Input: part model. Units: mm. Frame: model coordinates. A direction names the side the tool comes from. Coordinates: 2 decimals unless noted, no trailing zeros. Order: outer loops, then holes, each group sorted by start corner. A loop starts at its lowest first (then second) coordinate and runs counter-clockwise, first axis right, second up.
from build123d import *

# Parameters (mm, degrees)
BOSS_EXTRUDE1_DEPTH = 48.12
SKETCH3_W           = 16
SKETCH3_H           = 28.73
CUT_EXTRUDE1_DEPTH  = 47.12
SKETCH4_W           = 0.5
SKETCH4_H           = 10
BOSS_EXTRUDE2_DEPTH = 3
SKETCH5_W           = 2
SKETCH5_H           = 22.73
BOSS_EXTRUDE3_DEPTH = 4
SKETCH6_W           = 1
SKETCH6_H           = 19.230578804
CUT_EXTRUDE2_DEPTH  = 1
FILLET1_R           = 1
FILLET2_R           = 1
FILLET3_R           = 1
FILLET4_R           = 1


with BuildPart() as part:
    # Sketch2 → Boss-Extrude1 (new body)
    with BuildSketch(Plane(origin=(0, 0, 0), x_dir=(0, 0, -1), z_dir=(1, 0, 0))):
        Polygon((-1238.520696333, 790.685360665), (-1238.520696333, 788.685360665), (-1221.520696333, 788.685360665), (-1221.520696333, 759.955360665), (-1238.520696333, 759.955360665), (-1238.520696333, 757.955360665), (-1240.520696333, 757.955360665), (-1240.520696333, 790.685360665), align=None)
    extrude(amount=-BOSS_EXTRUDE1_DEPTH)

    # Sketch3 → Cut-Extrude1 (cut)
    with BuildSketch(Plane.ZY.offset(48.12)):
        with Locations((1230.520696333, 774.320360665)):
            Rectangle(SKETCH3_W, SKETCH3_H)
    extrude(amount=-CUT_EXTRUDE1_DEPTH, mode=Mode.SUBTRACT)

    # Sketch4 → Boss-Extrude2 (add)
    with BuildSketch(Plane.ZY.offset(48.12)):
        with Locations((1222.270696333, 774.320360665)):
            Rectangle(SKETCH4_W, SKETCH4_H)
    extrude(amount=BOSS_EXTRUDE2_DEPTH)

    # Sketch5 → Boss-Extrude3 (add)
    with BuildSketch(Plane(origin=(0, 0, 0), x_dir=(0, 0, -1), z_dir=(1, 0, 0))):
        with Locations((-1238.520696333, 774.320360665)):
            Rectangle(SKETCH5_W, SKETCH5_H)
    extrude(amount=BOSS_EXTRUDE3_DEPTH)

    # Sketch6 → Cut-Extrude2 (cut)
    with BuildSketch(Plane.XY.offset(1239.520696333)):
        with Locations((2, 773.582614675)):
            Rectangle(SKETCH6_W, SKETCH6_H)
    extrude(amount=-CUT_EXTRUDE2_DEPTH, mode=Mode.SUBTRACT)

    # Fillet1
    fillet1_edges = [part.edges().sort_by_distance(p)[0] for p in [
        (0, 774.320360665, 1239.520696333),
    ]]
    fillet(fillet1_edges, radius=FILLET1_R - 0.0001)  # a hair under: the kernel refuses the full size

    # Fillet2
    fillet2_edges = [part.edges().sort_by_distance(p)[0] for p in [
        (0, 774.320360665, 1237.520696333),
    ]]
    fillet(fillet2_edges, radius=FILLET2_R)

    # Fillet3
    fillet3_edges = [part.edges().sort_by_distance(p)[0] for p in [
        (0, 785.685360665, 1238.520646333),
    ]]
    fillet(fillet3_edges, radius=FILLET3_R)

    # Fillet4
    fillet4_edges = [part.edges().sort_by_distance(p)[0] for p in [
        (0, 762.955360665, 1238.520646333),
    ]]
    fillet(fillet4_edges, radius=FILLET4_R)


solid = part.part
Item 1: Ray query, probe 1 along Z at (x, y) = (-27, 769.5); probe 2 along Z at (x, y) = (-3, 759); probe 3 along X at (y, z) = (777, 1227.25). Return the intervals inside material, ascending.
Response values:
probe 1: z = 1221.52 to 1222.52, 1238.52 to 1240.52
probe 2: z = 1238.52 to 1240.52
probe 3: x = -1 to 0
Item 2: Cut plane B-B on x = -9.5. Return loops of the section in (y, z).
Response values:
outline: (757.96, 1238.52) - (790.69, 1238.52) - (790.69, 1240.52) - (757.96, 1240.52) - close; (759.96, 1221.52) - (788.69, 1221.52) - (788.69, 1222.52) - (759.96, 1222.52) - close
Item 3: Access query for faces 1 (the face through (2, 785.685, 1239)), 2 (the face through (-1, 775, 1230)), 3 (the face through (2, 774, 1237.521)), 4 (the face through (-48.12, 775, 1240)). Directions: +Z, -Z, +X, -X, +Y, -Y. A direction counts if a zero-diameter tool reaches every point of the face in a straight line with its end or side. Return the directions, or none.
Response values:
face 1: +Z, -Z, +X, +Y
face 2: -X, +Y, -Y
face 3: -Z, +X, +Y, -Y
face 4: +Z, -X, +Y, -Y
Item 4: Pin query (flat end, axial travel): pin 1 Ø4 at (y, z) = (766, 1236.5) entering from +X; pin 2 Ø1 at (y, z) = (772, 1226.5) entering from +X; pin 3 Ø6 at (y, z) = (768, 1231) entering from -X; pin 4 Ø3 at (y, z) = (772.5, 1237.5) entering from -X. Return the tip coordinate at first contact, or that it passes through.
Response values:
pin 1: stops at x = 4
pin 2: stops at x = 0
pin 3: stops at x = -1
pin 4: stops at x = -48.12
Item 5: Draft query along Z for faces 5 (the face through (-24, 775, 1238.521)), 6 (the face through (-50, 774, 1222.021)), 7 (the face through (-17, 788.685, 1222)). Return one class per face: pulls with the +Z half, pulls with the -Z half, needs draft (parallel to the pull), parting line crosses it, or undercut.
Response values:
face 5: undercut
face 6: pulls with the -Z half
face 7: needs draft
Item 6: Cut plane C-C on z = 1235.75. Return loops of the section in (x, y).
Response values:
outline: (-1, 759.96) - (0, 759.96) - (0, 788.69) - (-1, 788.69) - close
